Can you work these out from the model? Positions are in its coordinate system, mm. A direction names the side the tool comes from. Give positions to 0.01 mm unless a question says otherwise; leave off trailing zeros. Loops run counter-clockwise (first coordinate to the right, second up) from the corner with the lowest first, then second, coordinate; pieces in that order, holes last. Notation, with made-up numbers: (-14.5, -26) - (1.5, -26) arc R29 ccw to (1.5, 8) - close; hole circle Ø1 at (63.25, 26.5). An arc over 180 degrees is marked (long way). Answer as a JSON object with one key per item and string values. Group by question number.
Item 1: Please list where these lines run through material, in increasing order: L1, parallel to Y at x = -5.5, z = 8.5; L2, parallel to Y at x = -23, z = 4; L3, parallel to X at y = -11.5, z = -1.
Item 2: Which directions (+Z, -Z, +X, -X, +Y, -Y) give clear straight access to the entire face, cutting with the end or side of a thin tool? Please do faces 1 (the cylindrical face through (-3.4, -12.49, -2.61)), 2 (the flat face through (0, 0, 0)).
Item 3: Will these pins go through, and if not, where does the flat tip stop? pin 1 (2 mm diameter, centred on x = -1.5, z = -7.5, fed in from -Y) (3 decimals); pin 2 (6 mm diameter, centred on x = -16, y = -7, fed in from -Z); pin 3 (10 mm diameter, centred on x = 15, z = -17.5, fed in from -Y).
Item 4: Suppose I cut it at C-C on y = -4.75. Write out the boundary of the cut face in (x, z).
Item 5: Suppose I cut it at D-D on y = -7.5. Write out the boundary of the cut face in (x, z).
from build123d import *

# Parameters (mm, degrees)
F0_R     = 25.1181711361
F0_R_2   = 20.4995111856
F1_DEPTH = 3
F0_R_3   = 15.560509686
F2_DEPTH = 6
F0_R_4   = 10.0770984701
F3_DEPTH = 9
F0_R_5   = 4.2848341216
F4_DEPTH = 12
F0_R_6   = 1.2539122761
F5_DEPTH = 13
F6_DEPTH = 13


# Not quite as in the source:
# - a fillet or chamfer that OpenCascade refuses, or shapes differently, is made with other operations: its cross-section is extruded or revolved along the edge and cut away or added


with BuildPart() as f1:
    # F0 (on Front) → F1 (new body)
    with BuildSketch(Plane.XZ):
        Circle(F0_R)
        Circle(F0_R_2, mode=Mode.SUBTRACT)
    extrude(amount=F1_DEPTH)

    # F0 (on Front) → F2 (join)
    with BuildSketch(Plane.XZ):
        Circle(F0_R_2)
        Circle(F0_R_3, mode=Mode.SUBTRACT)
    extrude(amount=F2_DEPTH)

    # F0 (on Front) → F3 (join)
    with BuildSketch(Plane.XZ):
        Circle(F0_R_3)
        Circle(F0_R_4, mode=Mode.SUBTRACT)
    extrude(amount=F3_DEPTH)

    # F0 (on Front) → F4 (join)
    with BuildSketch(Plane.XZ):
        Circle(F0_R_4)
        Circle(F0_R_5, mode=Mode.SUBTRACT)
    extrude(amount=F4_DEPTH)

    # F0 (on Front) → F5 (join)
    with BuildSketch(Plane.XZ):
        Circle(F0_R_5)
        Circle(F0_R_6, mode=Mode.SUBTRACT)
    extrude(amount=F5_DEPTH)

    # F0 (on Front) → F6 (join)
    with BuildSketch(Plane.XZ):
        Circle(F0_R_6)
    extrude(amount=F6_DEPTH)

    # F7: fillet of radius 5 on 4 edges, made by hand

    # F7_s1 → F7_t2 (revolve, cut)
    with BuildSketch(Plane.XY):
        with BuildLine():
            ThreePointArc((25.1181711361, 0), (23.2742082286, -2.1833001327), (20.5355954411, -3))
            Line((20.5355954411, -3), (25.1181711361, -3))
            Line((25.1181711361, -3), (25.1181711361, 0))
        make_face()
    revolve(axis=Axis((0, -3, 0), (0, -1, 0)), mode=Mode.SUBTRACT)

    # F7_s3 → F7_t4 (revolve, cut)
    with BuildSketch(Plane.XY):
        with BuildLine():
            ThreePointArc((20.4995111856, -3), (18.6555482782, -5.1833001327), (15.9169354907, -6))
            Line((15.9169354907, -6), (20.4995111856, -6))
            Line((20.4995111856, -6), (20.4995111856, -3))
        make_face()
    revolve(axis=Axis((0, -6, 0), (0, -1, 0)), mode=Mode.SUBTRACT)

    # F7_s5 → F7_t6 (revolve, cut)
    with BuildSketch(Plane.XY):
        with BuildLine():
            ThreePointArc((15.560509686, -6), (13.7165467785, -8.1833001327), (10.977933991, -9))
            Line((10.977933991, -9), (15.560509686, -9))
            Line((15.560509686, -9), (15.560509686, -6))
        make_face()
    revolve(axis=Axis((0, -9, 0), (0, -1, 0)), mode=Mode.SUBTRACT)

    # F7_s7 → F7_t8 (revolve, cut)
    with BuildSketch(Plane.XY):
        with BuildLine():
            ThreePointArc((10.0770984701, -9), (8.2331355627, -11.1833001327), (5.4945227752, -12))
            Line((5.4945227752, -12), (10.0770984701, -12))
            Line((10.0770984701, -12), (10.0770984701, -9))
        make_face()
    revolve(axis=Axis((0, -12, 0), (0, -1, 0)), mode=Mode.SUBTRACT)


solid = f1.part
Worked out:
{
 "1": {"L1": "y = -9 to 0", "L2": "y = -2.14 to 0", "L3": "x = -7.61 to 7.61"},
 "2": {"face 1": "-Y", "face 2": "+Z, -Z, +X, -X, +Y"},
 "3": {"pin 1": "stops at y = -11.865", "pin 2": "stops at z = -13.2", "pin 3": "stops at y = -5.52"},
 "4": {"outline": "circle Ø38.45 at (0, 0)"},
 "5": {"outline": "circle Ø29.1 at (0, 0)"}
}
